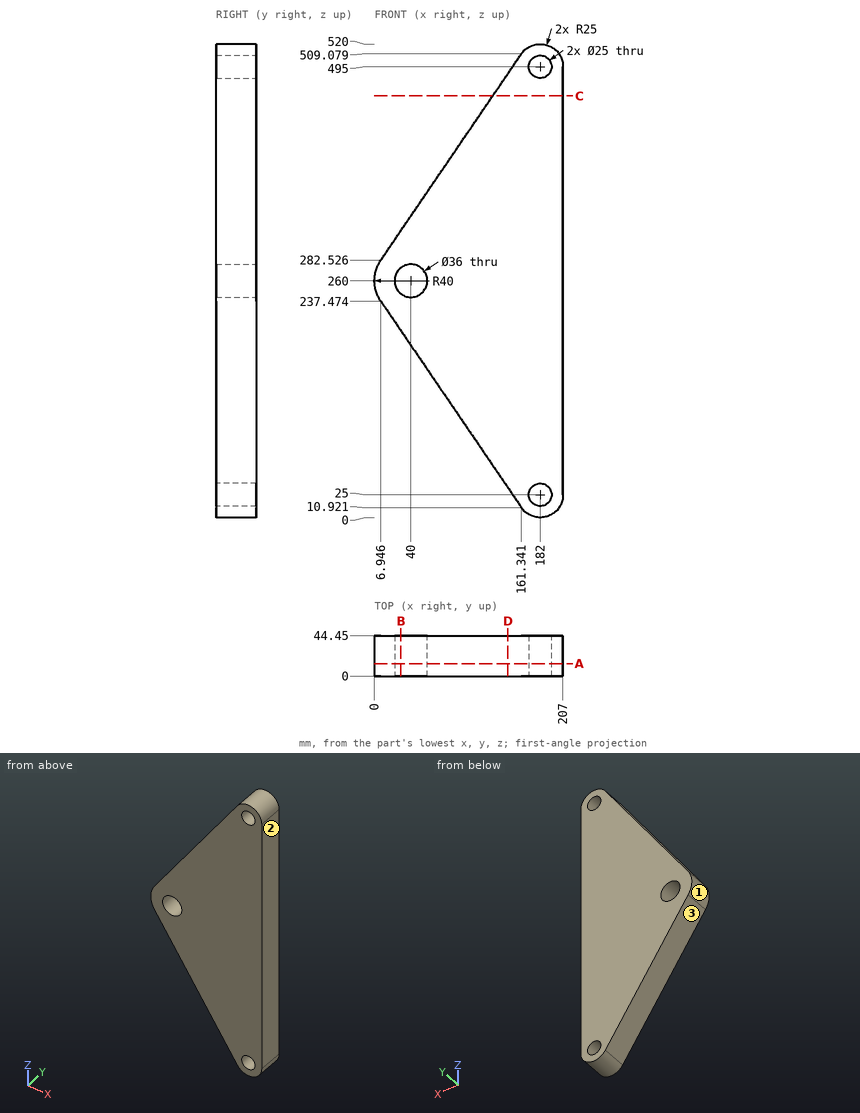
Part print with two shaded views. Sizes in mm from the minimum x, y, z corner. Coordinates: 2 decimals unless noted, no trailing zeros. Write each loop counter-clockwise with the first axis right and the second up, starting at its lowest first coordinate (ties: lowest second). Pieces come first, ordered by that corner, then holes. Notation, with made-up numbers: (48.5, 29) - (72.5, 29) arc R5 cw to (72.5, 37) - close; hole circle Ø1 at (85, 81). An arc over 180 degrees is marked (long way). Put each result on its own line as item: value.
1. Band-saw the part on B-B (x = 29). Write the cut outline in (y, z), then the cut area to 3 significant figures.
Final values:
outline: (0, 205.11) - (44.45, 205.11) - (44.45, 245.75) - (0, 245.75) - close; (0, 274.25) - (44.45, 274.25) - (44.45, 314.89) - (0, 314.89) - close
area: 3,610 mm²
2. Flat gauge pins, fed straight in: pin 1 Ø2 at (x, y) = (144, 7.5) entering from -Z; pin 2 Ø20 at (x, z) = (182, 25) entering from +Y; pin 3 Ø6 at (x, y) = (131, 11.5) entering from +Z; pin 4 Ø1.5 at (x, y) = (168, 16) entering from -Z. Where does each tip first touch, or does it go through?
Final values:
pin 1: stops at z = 34.9
pin 2: passes through
pin 3: stops at z = 468.96
pin 4: stops at z = 3.8
3. Band-saw the part on C-C (z = 463). Write the cut outline in (x, y), then the cut area to 3 significant figures.
Final values:
outline: (129.94, 0) - (207, 0) - (207, 44.45) - (129.94, 44.45) - close
area: 3,430 mm²
4. Band-saw the part on D-D (x = 146.5). Write the cut outline in (y, z).
Final values:
outline: (0, 32.7) - (44.45, 32.7) - (44.45, 487.3) - (0, 487.3) - close
5. Two-plate mould, pull along Z, no slides. Class the marked faces 1, 2 and 3: +Z half, -Z half, draft (parallel to the pull), parting line (faces both ways), or undercut.
Final values:
face 1: parting line
face 2: draft
face 3: -Z half
6. Probe line 1 along Z through (x, y) = (190, 13) (1 decimal); line 2 along X through (y, z) = (11.5, 27); line 3 along Z through (x, y) = (150.5, 2.5). List the from-to ranges inside material, lowest first. Write a range as [from, to].
Final values:
line 1: z = [1.3, 15.4], [34.6, 485.4], [504.6, 518.7]
line 2: x = [150.38, 169.66], [194.34, 207]
line 3: z = [26.83, 493.17]
7. Band-saw the part on A-A (y = 13.5). Write the cut outline in (x, z).
Final values:
outline: (6.95, 237.47) - (161.34, 10.92) arc R25 ccw to (207, 25) - (207, 495) arc R25 ccw to (161.34, 509.08) - (6.95, 282.53) arc R40 ccw to start; hole circle Ø36 at (40, 260); hole circle Ø25 at (182, 25); hole circle Ø25 at (182, 495)
